Verification items for the finished model (mm, model axes). Round coordinates to 2 decimals unless told otherwise and drop trailing zeros. Loops run counter-clockwise (first coordinate to the right, second up) from the corner with the lowest first, then second, coordinate; pieces in that order, holes last. Notation, with made-up numbers: (-18.75, 17.5) -> (-13.75, 17.5) arc R18 cw to (-13.75, 52.5) -> close; hole circle Ø1 at (40, 58.5). An arc over 180 degrees is marked (long way). Write item = value, one per line.
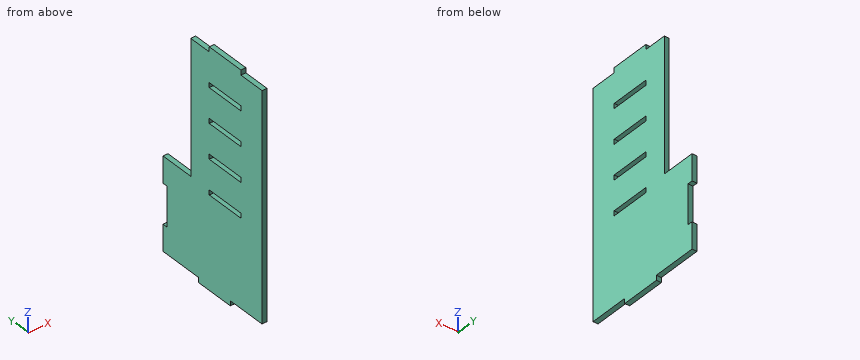
```python
from build123d import *

# Parameters (mm, degrees)
F0_W     = 152.4
F0_H     = 19.05
F1_DEPTH = 19.05


# Not quite as in the source:
# - a feature names something its author has since deleted; it is built from what else it names


with BuildPart() as f1:
    # F0 (on Right) → F1 (new body)
    with BuildSketch(Plane.YZ):
        Polygon((-69.85, 0), (-171.45, 0), (-171.45, -869.95), (-19.05, -869.95), (40.3552334547, -869.95), (133.35, -869.95), (171.45, -869.95), (171.45, -514.35), (171.45, 0), (82.55, 0), align=None)
        with Locations((6.35, -523.875)):
            Rectangle(F0_W, F0_H, mode=Mode.SUBTRACT)
        with Locations((6.35, -390.525)):
            Rectangle(F0_W, F0_H, mode=Mode.SUBTRACT)
        with Locations((6.35, -257.175)):
            Rectangle(F0_W, F0_H, mode=Mode.SUBTRACT)
        with Locations((6.35, -123.825)):
            Rectangle(F0_W, F0_H, mode=Mode.SUBTRACT)
        Polygon((40.3552334547, -869.95), (-19.05, -869.95), (-19.05, -889), (133.35, -889), (133.35, -869.95), align=None)
        Polygon((304.8, -514.35), (171.45, -514.35), (171.45, -869.95), (304.8, -869.95), (304.8, -768.35), (285.75, -768.35), (285.75, -615.95), (304.8, -615.95), align=None)
        with Locations((6.35, 9.525)):
            Rectangle(F0_W, F0_H)
    extrude(amount=F1_DEPTH)


solid = f1.part
```
(1) Sectioned sample at C-C, the plane z = -195.5. Record the cut outline in (x, y), and give its area (3 significant figures).
Filled sheet:
outline = (0, -171.45) -> (19.05, -171.45) -> (19.05, 171.45) -> (0, 171.45) -> close
area = 6,530 mm2
(2) Material ranges on probe 1 along Z at (x, y) = (9, 76); probe 2 along Z at (x, y) = (13, -29); probe 3 along Z at (x, y) = (5, 93), recorded low to high. Write a range as from..to.
Filled sheet:
probe_1 = -889..-533.4, -514.35..-400.05, -381..-266.7, -247.65..-133.35, -114.3..19.05
probe_2 = -869.95..-533.4, -514.35..-400.05, -381..-266.7, -247.65..-133.35, -114.3..19.05
probe_3 = -889..0
(3) Sectioned sample at B-B, the plane x = 12. Count the separate pieces of the cut face and the enclosed holes in it, and give its area (3 significant figures).
Filled sheet:
separate_pieces = 1
enclosed_holes = 4
area = 337,000 mm2
(4) Sectioned sample at D-D, the plane y = -27.5. Record the cut outline in (x, z), and give its area (3 significant figures).
Filled sheet:
outline = (0, -869.95) -> (19.05, -869.95) -> (19.05, -533.4) -> (0, -533.4) -> close; (0, -514.35) -> (19.05, -514.35) -> (19.05, -400.05) -> (0, -400.05) -> close; (0, -381) -> (19.05, -381) -> (19.05, -266.7) -> (0, -266.7) -> close; (0, -247.65) -> (19.05, -247.65) -> (19.05, -133.35) -> (0, -133.35) -> close; (0, -114.3) -> (19.05, -114.3) -> (19.05, 19.05) -> (0, 19.05) -> close
area = 15,500 mm2
(5) Sectioned sample at A-A, the plane y = 29. Record the cut outline in (x, z), and give its area (3 significant figures).
Filled sheet:
outline = (0, -889) -> (19.05, -889) -> (19.05, -533.4) -> (0, -533.4) -> close; (0, -514.35) -> (19.05, -514.35) -> (19.05, -400.05) -> (0, -400.05) -> close; (0, -381) -> (19.05, -381) -> (19.05, -266.7) -> (0, -266.7) -> close; (0, -247.65) -> (19.05, -247.65) -> (19.05, -133.35) -> (0, -133.35) -> close; (0, -114.3) -> (19.05, -114.3) -> (19.05, 19.05) -> (0, 19.05) -> close
area = 15,800 mm2
(6) Go/stop test with flat-tipped pins: pin 1 Ø5 at (x, y) = (4.5, -54.5) entering from -Z; pin 2 Ø8 at (x, z) = (14.5, -113.5) entering from +Y; pin 3 Ø5.5 at (x, z) = (8.5, -715.5) entering from +Y. Record where each tip stops, or that it passes through.
Filled sheet:
pin_1 = -869.95
pin_2 = 171.45
pin_3 = 285.75
